```python
from build123d import *
from OCP.BRepFilletAPI import BRepFilletAPI_MakeChamfer

# Parameters (mm, degrees)
SKETCH_1_W                         = 11.7
SKETCH_1_H                         = 12
EXTRUDE_1_DEPTH                    = 4.5
SKETCH_9_R                         = 3.5
EXTRUDE_2_DEPTH                    = 11.5
SKETCH_10_R                        = 1.75
EXTRUDE_3_DEPTH                    = 1.5
SKETCH_11_R                        = 3
EXTRUDE_4_DEPTH                    = 11.5
CHAMFER_1_SIZE                     = 1
CHAMFER_2_SIZE                     = 0.4
SKETCH_12_W                        = 6
SKETCH_12_H                        = 1.5
CUT_EXTRUDE_1_DEPTH                = 10
FILLET_1_R                         = 0.5
FILLET_2_R                         = 0.5
EXTRUDE_1_2_DEPTH                  = 1.25
CHAMFER_3_SIZE                     = 0.4
CHAMFER_3_SIZE2                    = 0.857802768
FILLET_3_R                         = 0.3
CHAMFER_3_OF_MIRROR_1_SIZE         = 0.4
CHAMFER_3_OF_MIRROR_1_SIZE2        = 0.857802768
FILLET_3_OF_MIRROR_1_R             = 0.3
EXTRUDE_2_2_DEPTH                  = 0.5
EXTRUDE_3_2_DEPTH                  = 0.75
FILLET_4_R                         = 0.5
PATTERN_LINEAR_1_COUNT             = 2
PATTERN_LINEAR_1_PITCH             = 2.5
FILLET_4_OF_PATTERN_LINEAR_1_R     = 0.5
PATTERN_LINEAR_1_COL_COUNT         = 2
PATTERN_LINEAR_1_COL_PITCH         = 2.5
FILLET_4_OF_PATTERN_LINEAR_1_COL_R = 0.5
EXTRUDE_START                      = 2.5
EXTRUDE_4_2_DEPTH                  = 0.5
EXTRUDE_5_DEPTH                    = 0.75
FILLET_5_R                         = 0.5
FILLET_5_OF_MIRROR_2_R             = 0.5


with BuildPart() as part:
    # Эскиз1 → Extrude 1 (new body)
    with BuildSketch(Plane(origin=(0, 0, 0), x_dir=(1, 0, 0), z_dir=(0, 1, 0))):
        Rectangle(SKETCH_1_W, SKETCH_1_H)
    extrude(amount=EXTRUDE_1_DEPTH)

    # Эскиз9 → Extrude 2 (add)
    with BuildSketch(Plane(origin=(0, 0, 0), x_dir=(1, 0, 0), z_dir=(0, 1, 0))):
        with Locations(Location((0, 0, 0), (0, 0, 270))):
            Circle(SKETCH_9_R)
    extrude(amount=EXTRUDE_2_DEPTH)

    # Эскиз10 → Extrude 3 (add)
    with BuildSketch(Plane(origin=(0, 11.5, 0), x_dir=(1, 0, 0), z_dir=(0, 1, 0))):
        with Locations(Location((0, 0, 0), (0, 0, 270))):
            Circle(SKETCH_10_R)
    extrude(amount=EXTRUDE_3_DEPTH)

    # Эскиз11 → Extrude 4 (add)
    with BuildSketch(Plane(origin=(0, 13, 0), x_dir=(1, 0, 0), z_dir=(0, 1, 0))):
        with Locations(Location((0, 0, 0), (0, 0, 270))):
            Circle(SKETCH_11_R)
    extrude(amount=EXTRUDE_4_DEPTH)

    # Фаска1
    chamfer_1_edges = [part.edges().sort_by_distance(p)[0] for p in [
        (0, 24.5, -3),
    ]]
    chamfer(chamfer_1_edges, length=CHAMFER_1_SIZE)

    # Фаска2
    chamfer_2_edges = [part.edges().sort_by_distance(p)[0] for p in [
        (0, 11.5, -3.5),
    ]]
    chamfer(chamfer_2_edges, length=CHAMFER_2_SIZE)

    # Эскиз12 → Вырез-Вытянуть1 (cut)
    with BuildSketch(Plane(origin=(0, 24.5, 0), x_dir=(1, 0, 0), z_dir=(0, 1, 0))):
        with Locations((0, 2.25)):
            Rectangle(SKETCH_12_W, SKETCH_12_H)
    extrude(amount=-CUT_EXTRUDE_1_DEPTH, mode=Mode.SUBTRACT)

    # Скругление1
    fillet_1_edges = [part.edges().sort_by_distance(p)[0] for p in [
        (0, 4.5, -3.5),
    ]]
    fillet(fillet_1_edges, radius=FILLET_1_R)

    # Скругление2
    fillet_2_edges = [part.edges().sort_by_distance(p)[0] for p in [
        (5.85, 2.25, 6),
        (-5.85, 2.25, 6),
        (-5.85, 2.25, -6),
        (5.85, 2.25, -6),
    ]]
    fillet(fillet_2_edges, radius=FILLET_2_R)

    # Эскиз13 → Extrude 1 2 (add, symmetric)
    with BuildSketch(Plane.XY):
        with BuildLine():
            Line((-5.85, 0), (-5.85, -1.129843788))
            ThreePointArc((-5.85, -1.129843788), (-5.861274336, -1.196045176), (-5.893826238, -1.254782798))
            Line((-5.893826238, -1.254782798), (-6.234378942, -1.680473678))
            ThreePointArc((-6.234378942, -1.680473678), (-6.358875719, -1.964024187), (-6.325398516, -2.271887168))
            Line((-6.325398516, -2.271887168), (-5.85, -3.5))
            Line((-5.85, -3.5), (-5.476972761, -3.355602359))
            Line((-5.476972761, -3.355602359), (-5.952371276, -2.127489527))
            ThreePointArc((-5.952371276, -2.127489527), (-5.963530344, -2.024868533), (-5.922031419, -1.930351697))
            Line((-5.922031419, -1.930351697), (-5.581478714, -1.504660817))
            ThreePointArc((-5.581478714, -1.504660817), (-5.483823009, -1.328447953), (-5.45, -1.129843788))
            Line((-5.45, -1.129843788), (-5.45, 0))
            Line((-5.45, 0), (-5.85, 0))
        make_face()
    extrude_1_2 = extrude(amount=EXTRUDE_1_2_DEPTH, both=True)

    # Фаска3: one chamfer whose edges measure the first distance from different faces: ONE call of the kernel's chamfer builder (chamfer() names one face for all edges)
    chamfer_3_edges_1 = [part.edges().sort_by_distance(p)[0] for p in [
        (-5.66348638, -3.427801179, 1.25),
    ]]
    chamfer_3_side_1 = [part.faces().sort_by_distance(p)[0] for p in [
        (-5.837614818, -1.735838174, 1.25),
    ]]
    chamfer_3_edges_2 = [part.edges().sort_by_distance(p)[0] for p in [
        (-5.66348638, -3.427801179, -1.25),
    ]]
    chamfer_3_side_2 = [part.faces().sort_by_distance(p)[0] for p in [
        (-5.837614818, -1.735838174, -1.25),
    ]]
    chamfer_3 = BRepFilletAPI_MakeChamfer(part.part.solid().wrapped)
    for e in chamfer_3_edges_1:
        chamfer_3.Add(CHAMFER_3_SIZE, CHAMFER_3_SIZE2, e.wrapped, chamfer_3_side_1[0].wrapped)  # the first distance lies on this face
    for e in chamfer_3_edges_2:
        chamfer_3.Add(CHAMFER_3_SIZE, CHAMFER_3_SIZE2, e.wrapped, chamfer_3_side_2[0].wrapped)  # the first distance lies on this face
    add(Compound.cast(chamfer_3.Shape()), mode=Mode.REPLACE)

    # Скругление3
    fillet_3_edges = [part.edges().sort_by_distance(p)[0] for p in [
        (-5.807884021, -3.05477394, -1.25),
        (-5.66348638, -3.427801179, 0.392197232),
        (-5.66348638, -3.427801179, -0.392197232),
        (-5.807884021, -3.05477394, 1.25),
    ]]
    fillet(fillet_3_edges, radius=FILLET_3_R)

    # Зеркальное отражение1: Extrude 1 2 across plane
    add(extrude_1_2.mirror(Plane(origin=(0, 0, 0), x_dir=(0, 0, 1), z_dir=(1, 0, 0))))

    # Фаска3 of Зеркальное отражение1: one chamfer whose edges measure the first distance from different faces: ONE call of the kernel's chamfer builder (chamfer() names one face for all edges)
    chamfer_3_of_mirror_1_edges_1 = [part.edges().sort_by_distance(p)[0] for p in [
        (5.66348638, -3.427801179, 1.25),
    ]]
    chamfer_3_of_mirror_1_side_1 = [part.faces().sort_by_distance(p)[0] for p in [
        (5.837614818, -1.735838174, 1.25),
    ]]
    chamfer_3_of_mirror_1_edges_2 = [part.edges().sort_by_distance(p)[0] for p in [
        (5.66348638, -3.427801179, -1.25),
    ]]
    chamfer_3_of_mirror_1_side_2 = [part.faces().sort_by_distance(p)[0] for p in [
        (5.837614818, -1.735838174, -1.25),
    ]]
    chamfer_3_of_mirror_1 = BRepFilletAPI_MakeChamfer(part.part.solid().wrapped)
    for e in chamfer_3_of_mirror_1_edges_1:
        chamfer_3_of_mirror_1.Add(CHAMFER_3_OF_MIRROR_1_SIZE, CHAMFER_3_OF_MIRROR_1_SIZE2, e.wrapped, chamfer_3_of_mirror_1_side_1[0].wrapped)  # the first distance lies on this face
    for e in chamfer_3_of_mirror_1_edges_2:
        chamfer_3_of_mirror_1.Add(CHAMFER_3_OF_MIRROR_1_SIZE, CHAMFER_3_OF_MIRROR_1_SIZE2, e.wrapped, chamfer_3_of_mirror_1_side_2[0].wrapped)  # the first distance lies on this face
    add(Compound.cast(chamfer_3_of_mirror_1.Shape()), mode=Mode.REPLACE)

    # Скругление3 of Зеркальное отражение1
    fillet_3_of_mirror_1_edges = [part.edges().sort_by_distance(p)[0] for p in [
        (5.807884021, -3.05477394, -1.25),
        (5.66348638, -3.427801179, 0.392197232),
        (5.66348638, -3.427801179, -0.392197232),
        (5.807884021, -3.05477394, 1.25),
    ]]
    fillet(fillet_3_of_mirror_1_edges, radius=FILLET_3_OF_MIRROR_1_R)

    # Эскиз14 → Extrude 2 2 (add, symmetric)
    with BuildSketch(Plane(origin=(0, 0, 0), x_dir=(0, 0, -1), z_dir=(1, 0, 0))):
        with BuildLine():
            Line((6, 0.85), (7.05, 0.85))
            ThreePointArc((7.05, 0.85), (7.262132034, 0.762132034), (7.35, 0.55))
            Line((7.35, 0.55), (7.35, -3.5))
            Line((7.35, -3.5), (7.65, -3.5))
            Line((7.65, -3.5), (7.65, 0.55))
            ThreePointArc((7.65, 0.55), (7.474264069, 0.974264069), (7.05, 1.15))
            Line((7.05, 1.15), (6, 1.15))
            Line((6, 1.15), (6, 0.85))
        make_face()
    extrude_2_2 = extrude(amount=EXTRUDE_2_2_DEPTH, both=True)

    # Эскиз15 → Extrude 3 2 (add, symmetric)
    with BuildSketch(Plane(origin=(0, 0, 0), x_dir=(0, 0, -1), z_dir=(1, 0, 0))):
        with BuildLine():
            Line((6, 0.85), (7.05, 0.85))
            ThreePointArc((7.05, 0.85), (7.262132034, 0.762132034), (7.35, 0.55))
            Line((7.35, 0.55), (7.35, 0))
            Line((7.35, 0), (7.65, 0))
            Line((7.65, 0), (7.65, 0.55))
            ThreePointArc((7.65, 0.55), (7.474264069, 0.974264069), (7.05, 1.15))
            Line((7.05, 1.15), (6, 1.15))
            Line((6, 1.15), (6, 0.85))
        make_face()
    extrude_3_2 = extrude(amount=EXTRUDE_3_2_DEPTH, both=True)

    # Скругление4
    fillet_4_edges = [part.edges().sort_by_distance(p)[0] for p in [
        (-0.5, -3.5, -7.5),
        (0.5, -3.5, -7.5),
    ]]
    fillet(fillet_4_edges, radius=FILLET_4_R - 0.0001)  # a hair under: the kernel refuses the full size

    # Линейный массив1: Extrude 2 2, Extrude 3 2 ×2
    with Locations(*[(i * PATTERN_LINEAR_1_PITCH, 0, 0) for i in range(1, PATTERN_LINEAR_1_COUNT)]):
        add(extrude_2_2)
        add(extrude_3_2)

    # Скругление4 of Линейный массив1
    fillet_4_of_pattern_linear_1_edges = [part.edges().sort_by_distance(p)[0] for p in [
        (2, -3.5, -7.5),
        (3, -3.5, -7.5),
    ]]
    fillet(fillet_4_of_pattern_linear_1_edges, radius=FILLET_4_OF_PATTERN_LINEAR_1_R - 0.0001)  # a hair under: the kernel refuses the full size

    # Линейный массив1 col: Extrude 2 2, Extrude 3 2 ×2
    with Locations(*[(-i * PATTERN_LINEAR_1_COL_PITCH, 0, 0) for i in range(1, PATTERN_LINEAR_1_COL_COUNT)]):
        add(extrude_2_2)
        add(extrude_3_2)

    # Скругление4 of Линейный массив1 col
    fillet_4_of_pattern_linear_1_col_edges = [part.edges().sort_by_distance(p)[0] for p in [
        (-3, -3.5, -7.5),
        (-2, -3.5, -7.5),
    ]]
    fillet(fillet_4_of_pattern_linear_1_col_edges, radius=FILLET_4_OF_PATTERN_LINEAR_1_COL_R - 0.0001)  # a hair under: the kernel refuses the full size

    # Эскиз16 → Extrude 4 2 (add, symmetric)
    with BuildSketch(Plane(origin=(0, 0, 0), x_dir=(0, 0, -1), z_dir=(1, 0, 0)).offset(EXTRUDE_START)):
        with BuildLine():
            Line((-6, 1.15), (-6.55, 1.15))
            ThreePointArc((-6.55, 1.15), (-6.974264069, 0.974264069), (-7.15, 0.55))
            Line((-7.15, 0.55), (-7.15, -3.5))
            Line((-7.15, -3.5), (-6.85, -3.5))
            Line((-6.85, -3.5), (-6.85, 0.55))
            ThreePointArc((-6.85, 0.55), (-6.762132034, 0.762132034), (-6.55, 0.85))
            Line((-6.55, 0.85), (-6, 0.85))
            Line((-6, 0.85), (-6, 1.15))
        make_face()
    extrude_4_2 = extrude(amount=EXTRUDE_4_2_DEPTH, both=True)

    # Эскиз17 → Вытянуть-Тонкостенный5 (add, symmetric)
    with BuildSketch(Plane(origin=(0, 0, 0), x_dir=(0, 0, -1), z_dir=(1, 0, 0)).offset(EXTRUDE_START)):
        with BuildLine():
            Line((-6, 1.15), (-6.55, 1.15))
            ThreePointArc((-6.55, 1.15), (-6.974264069, 0.974264069), (-7.15, 0.55))
            Line((-7.15, 0.55), (-7.15, 0))
            Line((-7.15, 0), (-6.85, 0))
            Line((-6.85, 0), (-6.85, 0.55))
            ThreePointArc((-6.85, 0.55), (-6.762132034, 0.762132034), (-6.55, 0.85))
            Line((-6.55, 0.85), (-6, 0.85))
            Line((-6, 0.85), (-6, 1.15))
        make_face()
    extrude_5 = extrude(amount=EXTRUDE_5_DEPTH, both=True)

    # Скругление5
    fillet_5_edges = [part.edges().sort_by_distance(p)[0] for p in [
        (3, -3.5, 7),
        (2, -3.5, 7),
    ]]
    fillet(fillet_5_edges, radius=FILLET_5_R - 0.0001)  # a hair under: the kernel refuses the full size

    # Зеркальное отражение2: Extrude 4 2, Вытянуть-Тонкостенный5 across plane
    add(extrude_4_2.mirror(Plane(origin=(0, 0, 0), x_dir=(0, 0, 1), z_dir=(1, 0, 0))))
    add(extrude_5.mirror(Plane(origin=(0, 0, 0), x_dir=(0, 0, 1), z_dir=(1, 0, 0))))

    # Скругление5 of Зеркальное отражение2
    fillet_5_of_mirror_2_edges = [part.edges().sort_by_distance(p)[0] for p in [
        (-3, -3.5, 7),
        (-2, -3.5, 7),
    ]]
    fillet(fillet_5_of_mirror_2_edges, radius=FILLET_5_OF_MIRROR_2_R - 0.0001)  # a hair under: the kernel refuses the full size


solid = part.part
```
Part model, mm, in its own coordinate system. A direction names the side the tool comes from. Round coordinates to 2 decimals unless told otherwise and drop trailing zeros. Write each loop counter-clockwise with the first axis right and the second up, starting at its lowest first coordinate (ties: lowest second). Pieces come first, ordered by that corner, then holes. Notation, with made-up numbers: M -17.75,56.5 L 22.25,56.5 A11 cw 22.25,64.5 Z; hole C 88,-37 d7. An arc over 180 degrees is marked long. Answer as CSV lines item,"result". Start each with the question number.
1) Drill centre lines: L1, parallel to X at y = 21.75, z = 0; L2, parallel to Y at x = -0.25, z = -4.75; L3, parallel to Z at x = -5.25, y = 1.5. Where is each one in solid material? Low to high.
2) Mould opens along X. For faces 1 (the face through (5.71, -2.75, 0.02)), 2 (the face through (-4, 4.5, -1.4)), 3 (the face through (6.09, -2.88, 0.02)) say: +X half, -X half, draft (parallel to the pull), parting line (faces both ways), or undercut.
3) Band-saw the part on A-A (y = 1.75). List the corners of the cut face in (x, z), then the cut area to 3 significant figures.
4) Band-saw the part on C-C (x = 5). List the corners of the cut face in (y, z), then the cut area to 3 significant figures.
5) Which spindle directions (+Z, -Z, +X, -X, +Y, -Y) get a long thin tool onto all of the face, cutting with end or side? Do faces 4 (the face through (5.8, -1.5, 1.25)), 5 (the face through (-2.5, 0.85, -6.5)), 6 (the face through (0, 1.15, -6.5)), 7 (the face through (5.8, -1.5, -1.25)), 8 (the face through (-5.85, 2, 0)). Say none if no direction does.
6) Band-saw the part on D-D (y = 7.75). List the corners of the cut face in (x, z).
7) Band-saw the part on B-B (z = 5). List the corners of the cut face in (x, y).
8) Drop flat-ended pins along their axis: pin 1 (1.6 mm diameter, centred on x = 0.5, y = -2.5, fed in from +Z); pin 2 (0.8 mm diameter, centred on x = 0.5, z = -6.5, fed in from -Y); pin 3 (0.5 mm diameter, centred on x = -2.5, z = -6.5, fed in from +Y). Give the stop position or say it passes through.
Worked out:
1,L1,"-3 to 3"
1,L2,"0 to 4.5"
1,L3,"-6 to 6"
2,face 1,"undercut"
2,face 2,"draft"
2,face 3,"+X half"
3,outline,"M -5.85,-5.5 A0.5 ccw -5.35,-6 L 5.35,-6 A0.5 ccw 5.85,-5.5 L 5.85,5.5 A0.5 ccw 5.35,6 L -5.35,6 A0.5 ccw -5.85,5.5 Z"
3,area,"140 mm²"
4,outline,"M 0,-6 L 4.5,-6 L 4.5,6 L 0,6 Z"
4,area,"54.0 mm²"
5,face 4,"+Z, +X, -X, -Y"
5,face 5,"+X, -X, -Y"
5,face 6,"-Z, +X, -X, +Y"
5,face 7,"-Z, +X, -X, -Y"
5,face 8,"+Z, -Z, -X, +Y"
6,outline,"C 0,0 d7"
7,outline,"M -5.85,0 L 5.85,0 L 5.85,4.5 L -5.85,4.5 Z"
8,pin 1,"z = -7.35"
8,pin 2,"y = 0.85"
8,pin 3,"y = 1.15"
